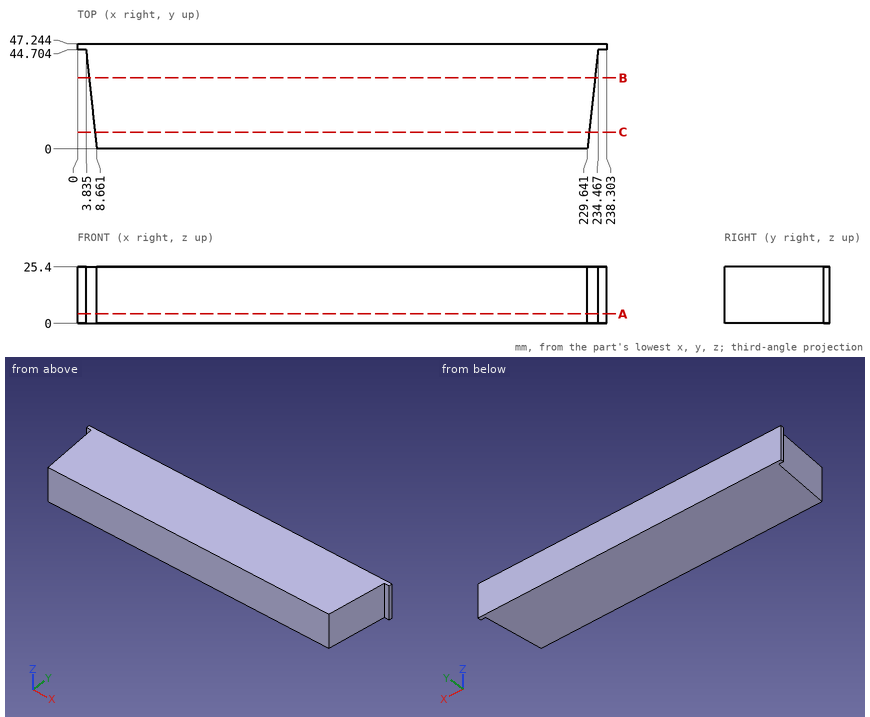
Job drawing, mm, ordinate dimensions from the low corner. One solid piece. Round coordinates to 2 decimals unless told otherwise and drop trailing zeros. Order: outer loops, then holes, each group sorted by start corner. A loop starts at its lowest first (then second) coordinate and runs counter-clockwise, first axis right, second up. Notation, with made-up numbers: (-32, 32.25) - (12, 32.25) arc R34 cw to (12, 71.25) - close; hole circle Ø1 at (55.25, -22.75). An arc over 180 degrees is marked (long way). Use CSV: the item, a comma, the result in double quotes. Start each with the question number.
1) Wall check: L1, parallel to X at y = 27, z = 15.75; L2, parallel to X at y = 40, z = 21.5. Give the ranges that are in metal, low to high. Write a range as [from, to].
2) Saw through at A-A (z = 4.25). List the corners of the cut face in (x, y) (1 decimal), and give its area (3 significant figures).
3) Pin check, flat tip, straight feed: pin 1 Ø2 at (y, z) = (37, 14) entering from +X. Stop position of the tip, or through.
4) Saw through at B-B (y = 32). List the corners of the cut face in (x, z).
5) Saw through at C-C (y = 7.5). List the corners of the cut face in (x, z), and give its area (3 significant figures).
Values follow:
1,L1,"x = [5.75, 232.56]"
1,L2,"x = [4.34, 233.96]"
2,outline,"(0, 44.7) - (3.8, 44.7) - (8.7, 0) - (229.6, 0) - (234.5, 44.7) - (238.3, 44.7) - (238.3, 47.2) - (0, 47.2) - close"
2,area,"10,700 mm2"
3,pin 1,"stops at x = 233.74"
4,outline,"(5.21, 0) - (233.1, 0) - (233.1, 25.4) - (5.21, 25.4) - close"
5,outline,"(7.85, 0) - (230.45, 0) - (230.45, 25.4) - (7.85, 25.4) - close"
5,area,"5,650 mm2"
